from build123d import *

# Parameters (mm, degrees)
SKETCH_W        = 53
SKETCH_H        = 86
PAD_DEPTH       = 30
POCKET_DEPTH    = 30
POCKET001_DEPTH = 30
POCKET002_DEPTH = 30
POCKET003_DEPTH = 30
POCKET004_DEPTH = 30
FILLET_R        = 8


with BuildPart() as part:
    # Sketch → Pad (new body)
    with BuildSketch(Plane.XY):
        Rectangle(SKETCH_W, SKETCH_H)
    extrude(amount=PAD_DEPTH)

    # Sketch001 (on Face6 of Pad) → Pocket (cut)
    with BuildSketch(Plane.XY.offset(30)):
        with BuildLine():
            ThreePointArc((16.5, 16.5), (0, 33), (-16.5, 16.5))
            Line((-16.5, -16.499996), (-16.5, 16.5))
            ThreePointArc((-16.5, -16.499996), (0, -33), (16.5, -16.499996))
            Line((26.5, -16.499996), (16.5, -16.499996))
            Line((26.5, 16.5), (26.5, -16.499996))
            Line((16.5, 16.5), (26.5, 16.5))
        make_face()
    extrude(amount=-POCKET_DEPTH, mode=Mode.SUBTRACT)

    # Sketch002 (on Face5 of Pocket) → Pocket001 (cut)
    with BuildSketch(Plane.XY.offset(30)):
        with BuildLine():
            ThreePointArc((0, 43), (-18.73833, 35.23833), (-26.5, 16.5))
            Line((-26.5, 16.5), (-26.5, 43))
            Line((-26.5, 43), (0, 43))
        make_face()
    extrude(amount=-POCKET001_DEPTH, mode=Mode.SUBTRACT)

    # Sketch003 (on Face4 of Pocket001) → Pocket002 (cut)
    with BuildSketch(Plane.XY.offset(30)):
        with BuildLine():
            ThreePointArc((26.5, 16.5), (18.73833, 35.23833), (0, 43))
            Line((0, 43), (26.5, 43))
            Line((26.5, 16.5), (26.5, 43))
        make_face()
    extrude(amount=-POCKET002_DEPTH, mode=Mode.SUBTRACT)

    # Sketch004 (on Face4 of Pocket002) → Pocket003 (cut)
    with BuildSketch(Plane.XY.offset(30)):
        with BuildLine():
            ThreePointArc((-26.5, -16.5), (-18.738343, -35.238316), (-3.9e-05, -43))
            Line((-3.9e-05, -43), (-26.5, -43))
            Line((-26.5, -16.5), (-26.5, -43))
        make_face()
    extrude(amount=-POCKET003_DEPTH, mode=Mode.SUBTRACT)

    # Sketch005 (on Face4 of Pocket003) → Pocket004 (cut)
    with BuildSketch(Plane.XY.offset(30)):
        with BuildLine():
            ThreePointArc((3.9e-05, -43), (18.738343, -35.238316), (26.5, -16.5))
            Line((26.5, -16.5), (26.5, -43))
            Line((26.5, -43), (3.9e-05, -43))
        make_face()
    extrude(amount=-POCKET004_DEPTH, mode=Mode.SUBTRACT)

    # Fillet
    fillet_edges = [part.edges().sort_by_distance(p)[0] for p in [
        (-16.5, 2e-06, 30),
    ]]
    fillet(fillet_edges, radius=FILLET_R)


solid = part.part
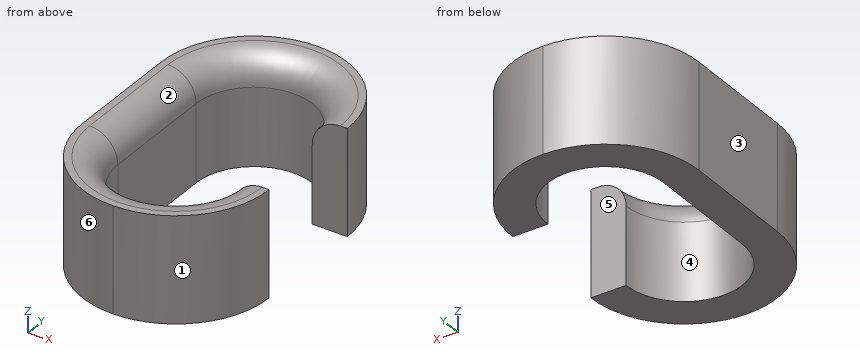
CAD build for the part. Positions are in the model's coordinates, mm. Face numbers are marked on the shaded views. A direction names the side the tool comes from. Give positions to 0.01 mm unless a question says otherwise; leave off trailing zeros. Write each loop counter-clockwise with the first axis right and the second up, starting at its lowest first coordinate (ties: lowest second). Pieces come first, ordered by that corner, then holes. Notation, with made-up numbers: M 48,60.25 L 78,60.25 A29 cw 78,89.25 Z; hole C -35.5,-31.75 d11. An arc over 180 degrees is marked long. Put each result on its own line as item: value. Start each with the question number.
(1) Mould opens along Y. For the marked faces 1, 2 and 3 say: +Y half, -Y half, draft (parallel to the pull), parting line (faces both ways), or undercut.
(2) Flat gauge pins, fed straight in: pin 1 Ø12 at (x, y) = (-8.5, -16.5) entering from +Z; pin 2 Ø5 at (x, z) = (23.5, 22) entering from -Y; pin 3 Ø1 at (x, z) = (3.5, 14) entering from +Y; pin 4 Ø17.5 at (y, z) = (5, 15.5) entering from +X. Where does each tip first touch, or does it go through?
(3) Which spindle directions (+Z, -Z, +X, -X, +Y, -Y) get a long thin tool onto all of the face, cutting with end or side? Do the marked faces 4, 5 and 6. Say none if no direction does.
(4) Probe L1, parallel to Y at x = 6.5, z = 10; L2, parallel to X at y = 22, z = 20.5; L3, parallel to X at y = -5.5, z = 20.5. List the from-to ranges inside material, lowest first.
(5) Band-saw the part on B-B, the plane y = -6.5. Write the cut outline in (x, z).
Response values:
1. face 1: -Y half
1. face 2: undercut
1. face 3: draft
2. pin 1: passes through
2. pin 2: stops at y = -32.66
2. pin 3: stops at y = 42.83
2. pin 4: stops at x = -16.5
3. face 4: +Z, -Z
3. face 5: +Z, -Z, +X
3. face 6: +Z, -Z, -X, -Y
4. L1: y = -42.19 to -31.67, 31.67 to 42.19
4. L2: x = -25.92 to -15.56, 15.56 to 25.92
4. L3: x = -26.5 to -16.5
5. outline: M -26.5,0 L -16.5,0 L -16.5,22 A8 ccw -24.5,30 L -26.5,30 Z
